```python
from build123d import *

# Parameters (mm, degrees)
BOSS_EXTRUDE1_START = 19
SKETCH1_R           = 4
SKETCH1_R_2         = 4.5
BOSS_EXTRUDE1_DEPTH = 1


with BuildPart() as part:
    # Sketch1 → Boss-Extrude1 (new body)
    with BuildSketch(Plane.XY.offset(BOSS_EXTRUDE1_START)):
        with BuildLine():
            Line((60.421564163, 1.006734174), (70, 0))
            Line((70, 0), (60.421564163, -1.006734174))
            ThreePointArc((60.421564163, -1.006734174), (54, -6.5), (47.578435837, -1.006734174))
            Line((47.578435837, -1.006734174), (7.205346635, -3.476058093))
            ThreePointArc((7.205346635, -3.476058093), (-8, 0), (7.205346635, 3.476058093))
            Line((7.205346635, 3.476058093), (47.578435837, 1.006734174))
            ThreePointArc((47.578435837, 1.006734174), (54, 6.5), (60.421564163, 1.006734174))
        make_face()
        with Locations((55, 0)):
            Circle(SKETCH1_R, mode=Mode.SUBTRACT)
        Circle(SKETCH1_R_2, mode=Mode.SUBTRACT)
    extrude(amount=BOSS_EXTRUDE1_DEPTH)


solid = part.part
```
Design review of the part built by this model. Coordinates are the model's own, in mm. A direction names the side the tool comes from. Coordinates: 2 decimals unless noted, no trailing zeros. Write each loop counter-clockwise with the first axis right and the second up, starting at its lowest first coordinate (ties: lowest second). Pieces come first, ordered by that corner, then holes.
1) Add section A-A (x = 0). Write out the cut boundary in (y, z), plus the area to 3 significant figures.
2) Add section D-D (x = 9). Write out the cut boundary in (y, z).
3) Insertion check: pin 1 (8 mm diameter, centred on x = 2, y = -2.5, fed in from -Z). The pin has a flat end and moves straight along its axis. Give the tip position at first contact, or say it passes through.
4) To check wall thickness, follow L1, parallel to Y at x = 0, z = 19.45; L2, parallel to X at y = 5.5, z = 19.95; L3, parallel to Y at x = -1, z = 19.9. State the ranges of each line that lie inside material, in increasing order.
5) Add section C-C (y = -5.5). Write out the cut boundary in (x, z), plus the area to 3 significant figures.
6) Add section B-B (z = 19.7). Write out the cut boundary in (x, y).
7) Machinability: for faces 1 (the flat face through (23, 0, 20)), 2 (the flat face through (27.11, 2.26, 19.49)), 3 (the flat face through (27.675, -2.224, 19.493)), which of the approach directions +Z, -Z, +X, -X, +Y, -Y give a long, thin tool a straight path to every point of the face, cutting with its end or side? Answer none if there is none.
Check result:
1. outline: (-8, 19) - (-4.5, 19) - (-4.5, 20) - (-8, 20) - close; (4.5, 19) - (8, 19) - (8, 20) - (4.5, 20) - close
1. area: 7.00 mm2
2. outline: (-3.37, 19) - (3.37, 19) - (3.37, 20) - (-3.37, 20) - close
3. pin 1: stops at z = 19
4. L1: y = -8 to -4.5, 4.5 to 8
4. L2: x = -5.81 to 5.81, 50.54 to 57.46
4. L3: y = -7.94 to -4.39, 4.39 to 7.94
5. outline: (-5.81, 19) - (5.81, 19) - (5.81, 20) - (-5.81, 20) - close; (50.54, 19) - (57.46, 19) - (57.46, 20) - (50.54, 20) - close
5. area: 18.5 mm2
6. outline: (7.21, -3.48) - (47.58, -1.01) arc R6.5 ccw to (60.42, -1.01) - (70, 0) - (60.42, 1.01) arc R6.5 ccw to (47.58, 1.01) - (7.21, 3.48) arc R8 ccw (long way) to start; hole circle Ø9 at (0, 0); hole circle Ø8 at (55, 0)
7. face 1: +Z, +X, -X, +Y, -Y
7. face 2: +Z, -Z, +Y
7. face 3: +Z, -Z, -Y
